Build history of the part. All positions in model axes, mm. A direction names the side the tool comes from. Coordinates: 2 decimals unless noted, no trailing zeros. Write each loop counter-clockwise with the first axis right and the second up, starting at its lowest first coordinate (ties: lowest second). Pieces come first, ordered by that corner, then holes.
```python
from build123d import *

# Parameters (mm, degrees)
BOSS_EXTRUDE1_DEPTH = 25.4
CUT_EXTRUDE2_START  = -12.192
CUT_EXTRUDE2_DEPTH  = 12.192
CUT_EXTRUDE3_DEPTH  = 141.749443769
SKETCH3_W           = 31.496
SKETCH3_H           = 6.096
CUT_EXTRUDE4_DEPTH  = 120.73640278
SKETCH4_R           = 3.96875
CUT_EXTRUDE5_DEPTH  = 163.137144219


# Read off the part's stored shape, not the designer's step: Cut-Extrude2
with BuildPart() as part:
    # Sketch1 → Boss-Extrude1 (new, symmetric)
    with BuildSketch(Plane.XY):
        Polygon((0, 0), (85.852, 0), (131.703269909, -45.851269909), (149.663782152, -27.890757667), (111.587496198, 10.185528286), (102.607240077, 1.205272165), (91.112512242, 12.7), (0, 12.7), align=None)
    extrude(amount=BOSS_EXTRUDE1_DEPTH, both=True)

    # Cut-Extrude2 outline → Cut-Extrude2 (cut)
    with BuildSketch(Plane(origin=(60.886512242, 60.886512242, 0), x_dir=(0, 0, -1), z_dir=(0.707106781186544, 0.7071067811865511, 0)).offset(CUT_EXTRUDE2_START)):
        with BuildLine():
            ThreePointArc((25.4, -119.183037491), (17.740042491, -122.543911277), (9.652, -124.677919317))
            Line((9.652, -124.677919317), (9.652, -71.702019136))
            Line((9.652, -71.702019136), (-9.652, -71.702019136))
            Line((-9.652, -71.702019136), (-9.652, -124.677919317))
            ThreePointArc((-9.652, -124.677919317), (-17.740042491, -122.543911277), (-25.4, -119.183037491))
            Line((-25.4, -119.183037491), (-25.4, -125.550019136))
            Line((-25.4, -125.550019136), (25.4, -125.550019136))
            Line((25.4, -125.550019136), (25.4, -119.183037491))
        make_face()
    extrude(amount=CUT_EXTRUDE2_DEPTH, mode=Mode.SUBTRACT)

    # Sketch2_5 → Cut-Extrude3 (cut, through all)
    with BuildSketch(Plane(origin=(60.886512242, 60.886512242, 0), x_dir=(0, 0, -1), z_dir=(0.707106781186544, 0.7071067811865511, 0))):
        with BuildLine():
            Line((-9.652, -124.677919317), (-9.652, -125.550019136))
            Line((-9.652, -125.550019136), (0, -125.550019136))
            ThreePointArc((0, -125.550019136), (-4.845659452, -125.331551005), (-9.652, -124.677919317))
        make_face()
        with BuildLine():
            Line((-25.4, -119.183037491), (-25.4, -125.550019136))
            Line((-25.4, -125.550019136), (-9.652, -125.550019136))
            Line((-9.652, -125.550019136), (-9.652, -124.677919317))
            ThreePointArc((-9.652, -124.677919317), (-17.740042491, -122.543911277), (-25.4, -119.183037491))
        make_face()
        with BuildLine():
            Line((9.652, -124.677919317), (9.652, -125.550019136))
            Line((9.652, -125.550019136), (25.4, -125.550019136))
            Line((25.4, -125.550019136), (25.4, -119.183037491))
            ThreePointArc((25.4, -119.183037491), (17.740042491, -122.543911277), (9.652, -124.677919317))
        make_face()
        with BuildLine():
            ThreePointArc((9.652, -124.677919317), (4.845659452, -125.331551005), (0, -125.550019136))
            Line((0, -125.550019136), (9.652, -125.550019136))
            Line((9.652, -125.550019136), (9.652, -124.677919317))
        make_face()
    extrude(amount=-CUT_EXTRUDE3_DEPTH, mode=Mode.SUBTRACT)

    # Sketch3 → Cut-Extrude4 (cut, through all)
    with BuildSketch(Plane(origin=(50.700983956, -50.700983956, 0), x_dir=(0, 0, 1), z_dir=(-0.7071067811865549, 0.7071067811865401, 0))):
        with Locations((0, 76.962531378)):
            Rectangle(SKETCH3_W, SKETCH3_H)
    extrude(amount=-CUT_EXTRUDE4_DEPTH, mode=Mode.SUBTRACT)

    # Sketch4 → Cut-Extrude5 (cut, through all)
    with BuildSketch(Plane(origin=(0, 12.7, 0), x_dir=(1, 0, 0), z_dir=(0, 1, 0))):
        with Locations(Location((15.748, 12.7, 0), (0, 0, 180))):
            Circle(SKETCH4_R)
        with Locations(Location((69.596, 12.7, 0), (0, 0, 180))):
            Circle(SKETCH4_R)
        with Locations(Location((15.748, -12.7, 0), (0, 0, 180))):
            Circle(SKETCH4_R)
        with Locations(Location((69.596, -12.7, 0), (0, 0, 180))):
            Circle(SKETCH4_R)
    extrude(amount=-CUT_EXTRUDE5_DEPTH, mode=Mode.SUBTRACT)


solid = part.part
```
1. Saw through at A-A on z = 11. List the corners of the cut face in (x, y) (1 decimal).
Computed values:
outline: (0, 0) - (12.2, 0) - (12.2, 12.7) - (0, 12.7) - close; (19.3, 0) - (66, 0) - (66, 12.7) - (19.3, 12.7) - close; (73.2, 0) - (85.9, 0) - (130.9, -45) - (140.2, -35.7) - (103, 1.6) - (102.6, 1.2) - (91.1, 12.7) - (73.2, 12.7) - close; (107.3, 5.9) - (144.6, -31.4) - (148.9, -27.1) - (111.6, 10.2) - close
2. Saw through at C-C on z = 3.5. List the corners of the cut face in (x, y), plus the area to 3 significant figures.
Computed values:
outline: (0, 0) - (85.85, 0) - (131.62, -45.77) - (140.96, -36.43) - (102.97, 1.56) - (102.61, 1.21) - (91.11, 12.7) - (0, 12.7) - close
area: 2,010 mm2
3. Mould opens along X. For faces 1 (the face through (88.4, -2.2, 25.4)), 2 (the face through (108.457, -22.605, 0.356)), 3 (the face through (96.94, 6.87, 0.36)) say: +X half, -X half, draft (parallel to the pull), parting line (faces both ways), or undercut.
Computed values:
face 1: draft
face 2: -X half
face 3: undercut
4. Saw through at B-B on y = -11. List the corners of the cut face in (x, z), plus the area to 3 significant figures.
Computed values:
outline: (96.85, -25.4) - (132.77, -25.4) - (132.77, -9.65) - (124.15, -9.65) - (124.15, -15.75) - (115.53, -15.75) - (115.53, 15.75) - (124.15, 15.75) - (124.15, 9.65) - (132.77, 9.65) - (132.77, 25.4) - (96.85, 25.4) - close
area: 1,390 mm2
5. Probe line 1 along X through (y, z) = (9, -12); line 2 along X through (y, z) = (5, -12); line 3 along Y through (x, z) = (63.5, -1). List the from-to ranges inside material, lowest first.
Computed values:
line 1: x = 0 to 11.84, 19.65 to 65.69, 73.5 to 94.81, 110.4 to 112.77
line 2: x = 0 to 11.84, 19.65 to 65.69, 73.5 to 98.81, 108.15 to 116.77
line 3: y = 0 to 12.7
6. 3-axis set-ups, long thin cutter, end or side, ignore diameter. For faces 4 (the face through (42, 0, 0)), 5 (the face through (121.74, -17.21, -0.22)), 6 (the face through (108.2, 6.8, -10.9)), 7 (the face through (128, -11, -9.652)): which of +Z, -Z, +X, -X, +Y, -Y reach the whole face in a straight line?
Computed values:
face 4: +Z, -Z, -X, -Y
face 5: none
face 6: +Z, -Z, +Y
face 7: +X, +Y
7. Flat gauge pins, fed straight in: pin 1 (8 mm diameter, centred on y = -14.5, z = -7, fed in from +X); pin 2 (1.5 mm diameter, centred on y = -29.5, z = -12.5, fed in from -X); pin 3 (1 mm diameter, centred on y = -9, z = -6.5, fed in from +X); pin 4 (12 mm diameter, centred on y = 0, z = 12.5, fed in from -X). Where does each tip first touch, or does it go through?
Computed values:
pin 1: stops at x = 139.27
pin 2: stops at x = 114.6
pin 3: stops at x = 114.03
pin 4: stops at x = 0
8. Saw through at D-D on x = 55.5. List the corners of the cut face in (y, z).
Computed values:
outline: (0, -25.4) - (12.7, -25.4) - (12.7, 25.4) - (0, 25.4) - close
